Here's how the part is built. I have some questions about the finished solid (model axes, mm). A direction names the side the tool comes from. Give positions to 0.01 mm unless a question says otherwise; leave off trailing zeros. Write each loop counter-clockwise with the first axis right and the second up, starting at its lowest first coordinate (ties: lowest second). Pieces come first, ordered by that corner, then holes. Notation, with made-up numbers: (-39, 38) - (-7, 38) arc R13 cw to (-7, 63) - close; hole circle Ø2 at (55, 65.5). An arc over 180 degrees is marked (long way). One line per item, written item: value. Start each with the question number.
1) Please list where these lines run through material, in increasing order: L1, parallel to Z at x = -60, y = 12.4; L2, parallel to Z at x = 60, y = 3.5; L3, parallel to X at y = 8, z = 1.25. Write a range as [from, to].
2) We'd pull the mould along Z, two halves only. Please class faces 1 (the flat face through (122, 9.7, 2)), 2 (the cylindrical face through (-122.08, 4.78, 0.86)), 3 (the flat face through (2, 0, 2)): +Z half, -Z half, draft (parallel to the pull), parting line (faces both ways), or undercut.
3) Imagine slicing it at B-B on z = 0. Count the separate pieces of the cut face and the enclosed holes in it, plus the area to 3 significant figures.
4) On a 3-axis mill with a long thin cutter (end or side, diameter ignored), from which of +Z, -Z, +X, -X, +Y, -Y can I reach the whole of each face in a straight line? I mean faces 4 (the flat face through (-130, 8, 0)), 5 (the flat face through (2, 9.7, 2)). Say none if no direction works.
5) Imagine slicing it at C-C on x = -94. Write out the boundary of the cut face in (y, z), plus the area to 3 significant figures.
6) I'm going to push flat-ended pins straight in: P1, Ø0.6, axis at x = -52, y = 7, coming from the -Z side; P2, Ø7, axis at x = -60, z = 0, coming from the +Y side; P3, Ø2, axis at x = 13, y = 7, coming from the +Z side. Where does each tip first touch, or does it pass through?
from build123d import *

# Parameters (mm, degrees)
EXTRUDE_1_DEPTH                  = 130
HOLE_WIZARD_M4_78051_D           = 4.5
HOLE_WIZARD_M4_78051_CBORE_D     = 7.5
HOLE_WIZARD_M4_78051_CBORE_DEPTH = 5.3
PATTERN_LINEAR_1_COUNT           = 3
PATTERN_LINEAR_1_PITCH           = 60
PATTERN_LINEAR_2_COUNT           = 3
PATTERN_LINEAR_2_PITCH           = 60


with BuildPart() as part:
    # Эскиз1 → Бобышка-Вытянуть1 (new, symmetric)
    with BuildSketch(Plane(origin=(0, 0, 0), x_dir=(0, 0, -1), z_dir=(1, 0, 0))):
        with BuildLine():
            Line((-7.5, 0.707106781), (-6.792893219, 0))
            Line((-6.792893219, 0), (6.792893219, 0))
            Line((6.792893219, 0), (7.5, 0.707106781))
            Line((7.5, 0.707106781), (7.5, 3.7))
            Line((7.5, 3.7), (4.8, 6.4))
            Line((4.8, 6.4), (4.8, 8.4))
            Line((4.8, 8.4), (5.21443454, 8.81443454))
            ThreePointArc((5.21443454, 8.81443454), (5.66862915, 9.73137085), (6.58556546, 10.18556546))
            Line((6.58556546, 10.18556546), (7.5, 11.1))
            Line((7.5, 11.1), (7.5, 12.5))
            Line((7.5, 12.5), (6.58556546, 13.41443454))
            ThreePointArc((6.58556546, 13.41443454), (5.66862915, 13.86862915), (5.21443454, 14.78556546))
            Line((5.21443454, 14.78556546), (5, 15))
            Line((5, 15), (-5, 15))
            Line((-5, 15), (-5.21443454, 14.78556546))
            ThreePointArc((-5.21443454, 14.78556546), (-5.66862915, 13.86862915), (-6.58556546, 13.41443454))
            Line((-6.58556546, 13.41443454), (-7.5, 12.5))
            Line((-7.5, 12.5), (-7.5, 11.1))
            Line((-7.5, 11.1), (-6.58556546, 10.18556546))
            ThreePointArc((-6.58556546, 10.18556546), (-5.66862915, 9.73137085), (-5.21443454, 8.81443454))
            Line((-5.21443454, 8.81443454), (-4.8, 8.4))
            Line((-4.8, 8.4), (-4.8, 6.4))
            Line((-4.8, 6.4), (-7.5, 3.7))
            Line((-7.5, 3.7), (-7.5, 0.707106781))
        make_face()
    extrude(amount=EXTRUDE_1_DEPTH, both=True)

    # Цековка M4 для болта с шестигранной головкой класса А ГОСТ 78051 (through all)
    with Locations(Plane(origin=(0, 15, 0), x_dir=(1, 0, 0), z_dir=(0, 1, 0))):
        with Locations((0, 0)):
            hole_wizard_m4_78051 = CounterBoreHole(HOLE_WIZARD_M4_78051_D / 2, HOLE_WIZARD_M4_78051_CBORE_D / 2, HOLE_WIZARD_M4_78051_CBORE_DEPTH)

    # Линейный массив1: Цековка M4 для болта с шестигранной головкой класса А ГОСТ 78051 ×3
    with Locations(*[(i * PATTERN_LINEAR_1_PITCH, 0, 0) for i in range(1, PATTERN_LINEAR_1_COUNT)]):
        add(hole_wizard_m4_78051, mode=Mode.SUBTRACT)

    # Линейный массив2: Цековка M4 для болта с шестигранной головкой класса А ГОСТ 78051 ×3
    with Locations(*[(-i * PATTERN_LINEAR_2_PITCH, 0, 0) for i in range(1, PATTERN_LINEAR_2_COUNT)]):
        add(hole_wizard_m4_78051, mode=Mode.SUBTRACT)


solid = part.part
Numbers:
1. L1: [-7.5, -3.75], [3.75, 7.5]
1. L2: [-7.5, -2.25], [2.25, 7.5]
1. L3: [-130, -121.87], [-118.13, -61.87], [-58.13, -1.87], [1.87, 58.13], [61.87, 118.13], [121.87, 130]
2. face 1: undercut
2. face 2: undercut
2. face 3: draft
3. separate pieces: 6
3. enclosed holes: 0
3. area: 3,480 mm^2
4. face 4: +Z, -Z, -X, +Y, -Y
4. face 5: +Y
5. outline: (0, -6.79) - (0.71, -7.5) - (3.7, -7.5) - (6.4, -4.8) - (8.4, -4.8) - (8.81, -5.21) arc R1.6 cw to (10.19, -6.59) - (11.1, -7.5) - (12.5, -7.5) - (13.41, -6.59) arc R1.6 cw to (14.79, -5.21) - (15, -5) - (15, 5) - (14.79, 5.21) arc R1.6 cw to (13.41, 6.59) - (12.5, 7.5) - (11.1, 7.5) - (10.19, 6.59) arc R1.6 cw to (8.81, 5.21) - (8.4, 4.8) - (6.4, 4.8) - (3.7, 7.5) - (0.71, 7.5) - (0, 6.79) - close
5. area: 191 mm^2
6. P1: z = -4.8
6. P2: y = 9.7
6. P3: z = 5.2
